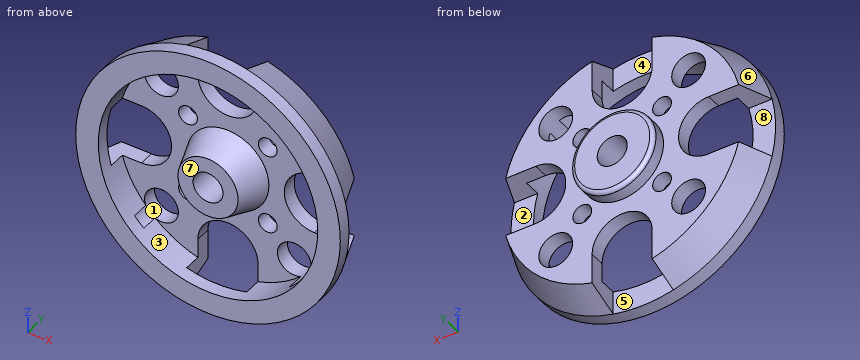
Autodesk Inventor part; units mm, degrees
ref_plane "YZ Plane" through (0, 0, 0) normal (1, 0, 0) x (0, 1, 0)
ref_plane "XZ Plane" through (0, 0, 0) normal (0, 1, 0) x (-1, 0, 0)
ref_plane "XY Plane" through (0, 0, 0) normal (0, 0, 1) x (1, 0, 0)
sketch "Sketch1" plane through (0, 0, 0) normal (0, 0, 1) x (1, 0, 0)
  line L0 (0, 0) -> (17.6, 0)
  line L1 (17.6, 0) -> (17.6, 6)
  line L2 (17.6, 6) -> (0, 6)
  line L3 (0, 6) -> (0, 0) construction
  line L4 (0, 6) -> (5.5, 6)
  line L5 (5.5, 6) -> (5.5, 8)
  line L6 (5.5, 8) -> (0, 8)
  line L7 (0, 8) -> (0, 6) construction
  line L8 (16, 6) -> (16, 0) construction
  line L9 (16, 6) -> (17.6, 1.75)
  line L10 (0, 0) -> (2, 0)
  line L11 (2, 0) -> (2, 8)
  line L12 (2, 8) -> (0, 8)
  line L13 (0, 8) -> (0, 0) construction
  dimension "d0" = 17.6
  dimension "d1" = 6
  dimension "d2" = 5.5
  dimension "d3" = 2
  dimension "d4" = 16
  dimension "d5" = 1.75
  dimension "d6" = 2
revolve "Revolution1" add sketch "Sketch1" angle 360 about axis through (0, 8, 0) along (0, -1, 0) contours L11 L2 L9 L1 L0 | L11 L6 L5 L2
sketch "Sketch2" plane through (0, 6, 0) normal (0, 1, 0) x (1, 0, 0)
  arc A0 (-11.5, -4) -> (-11.5, 4) centre (-11.5, 0) ccw
  circle A1 centre (0, 0) radius 11.5 construction
  line L0 (-11.5, 0) -> (0, 0) construction
  line L1 (-11.5, -4) -> (-21.025, -4)
  line L2 (-21.025, -4) -> (-21.025, 4)
  line L3 (-21.025, 4) -> (-11.5, 4)
  line L4 (-11.5, 4) -> (-11.5, -4) construction
  circle A2 centre (0, 0) radius 2
  circle A3 centre (0, 0) radius 7.5 construction
  circle A4 centre (0, 0) radius 12.5 construction
  line L5 (0, 0) -> (-8.8388, 8.8388) construction
  circle A5 centre (-5.3033, 5.3033) radius 1.25
  circle A6 centre (-8.8388, 8.8388) radius 2.25
  line L6 (-4, -11.5) -> (4, -11.5) construction
  line L7 (4, -11.5) -> (4, -21.025)
  line L8 (4, -21.025) -> (-4, -21.025)
  line L9 (-4, -21.025) -> (-4, -11.5)
  arc A7 (4, -11.5) -> (-4, -11.5) centre (0, -11.5) ccw
  circle A8 centre (-5.3033, -5.3033) radius 1.25
  circle A9 centre (-8.8388, -8.8388) radius 2.25
  line L10 (11.5, -4) -> (11.5, 4) construction
  line L11 (11.5, 4) -> (21.025, 4)
  line L12 (21.025, 4) -> (21.025, -4)
  line L13 (21.025, -4) -> (11.5, -4)
  arc A10 (11.5, 4) -> (11.5, -4) centre (11.5, 0) ccw
  circle A11 centre (5.3033, -5.3033) radius 1.25
  circle A12 centre (8.8388, -8.8388) radius 2.25
  line L14 (4, 11.5) -> (-4, 11.5) construction
  line L15 (-4, 11.5) -> (-4, 21.025)
  line L16 (-4, 21.025) -> (4, 21.025)
  line L17 (4, 21.025) -> (4, 11.5)
  arc A13 (-4, 11.5) -> (4, 11.5) centre (0, 11.5) ccw
  circle A14 centre (5.3033, 5.3033) radius 1.25
  circle A15 centre (8.8388, 8.8388) radius 2.25
  dimension "d9" = 23
  dimension "d11" = 15
  dimension "d12" = 25
  dimension "d8" = 8
  dimension "d10" = 9.525
  dimension "d13" = 45
  dimension "d14" = 2.5
  dimension "d15" = 4.5
  dimension "d18" = 360
extrude "Extrusion1" cut sketch "Sketch2" against normal blind 4.25
sketch "Sketch3" plane through (0, 0, 0) normal (0, -1, 0) x (1, 0, 0)
  circle A0 centre (0, 0) radius 2
  arc A1 (17.1394, 4) -> (4, 17.1394) centre (0, 0) ccw
  circle A2 centre (0, 0) radius 17.6
  circle A3 centre (0, 0) radius 14.6
  circle A4 centre (0, 0) radius 4
  dimension "d22" = 3
  dimension "d23" = 8
extrude "Extrusion2" cut sketch "Sketch3" against normal blind 4 contours A3
chamfer "Chamfer1" distance 4 angle 20 1 edges at (-4, 4, 0) measured on face at (3.987, 2.6667, -0.3219)
fillet "Fillet1" radius 0.5 1 edges at (-5.5, 8, 0)
properties part number "Top" material "Stainless Steel"
Read the model definition and answer for the solid it produces. Units are mm, in the model's axes. Face numbers are marked on the shaded views. A direction names the side the tool comes from. Coordinates: 2 decimals unless noted, no trailing zeros. Loops run counter-clockwise (first coordinate to the right, second up) from the corner with the lowest first, then second, coordinate; pieces in that order, holes last. Notation, with made-up numbers: (32, 89.5) -> (49, 89.5) arc R24 ccw to (49, 99.5) -> close; hole circle Ø7 at (11, 63.5). An arc over 180 degrees is marked (long way). Return JSON: item names as keys, results as strings.
Item 1: Find the intervals of material crossed by probe 1 along X at (y, z) = (4.5, -5); probe 2 along Z at (x, y) = (0, 5.5); probe 3 along Y at (x, z) = (7.5, -6.5), in increasing order.
Answers:
{"probe 1": "x = -15.79 to -6.52, -4.09 to 4.09, 6.52 to 15.79", "probe 2": "z = -7.5 to -2, 2 to 7.5", "probe 3": "y = 4 to 6"}
Item 2: Find section D-D (y = 6.5). Determine the outline of the cut face in (x, z).
Answers:
{"outline": "circle Ø11 at (0, 0); hole circle Ø4 at (0, 0)"}
Item 3: Find section C-C (y = 1). Determine the outline of the cut face in (x, z), plus the area to 3 significant figures.
Answers:
{"outline": "circle Ø35.2 at (0, 0); circle Ø8.73 at (0, 0); hole circle Ø29.2 at (0, 0); hole circle Ø4 at (0, 0)", "area": "351 mm2"}
Item 4: Find section A-A (z = 0). Count the separate pieces of the cut face and the enclosed holes in it, plus the area to 3 significant figures.
Answers:
{"separate pieces": "4", "enclosed holes": "0", "area": "68.2 mm2"}
Item 5: For a pull along Z with two mould halves and no side action, classify the marked faces 6, 7 and 8 as +Z half, -Z half, draft (parallel to the pull), parting line (faces both ways), or undercut.
Answers:
{"face 6": "+Z half", "face 7": "draft", "face 8": "undercut"}
Item 6: For the marked faces 1, 2, 3, 4 and 5, determine the directions among +Z, -Z, +X, -X, +Y, -Y from which every point of the face is accessible in a straight line to the end or side of a thin tool.
Answers:
{"face 1": "+Y", "face 2": "+X, +Y", "face 3": "-Y", "face 4": "+Z, +Y", "face 5": "-Z, +Y"}
Item 7: Flat-ended cylindrical pins translate along their axes: P1, Ø3, axis at x = 1, z = -15, coming from the +Y side; P2, Ø5, axis at x = 8.84, z = 8.84, coming from the +Y side; P3, Ø3, axis at y = 4, z = -1, coming from the +X side. Find the tip coordinate at first contact, or state that the pin passes through.
Answers:
{"P1": "stops at y = 1.75", "P2": "stops at y = 6", "P3": "stops at x = 8.38"}
